Design review of the part built by this model. Coordinates are the model's own, in mm. A direction names the side the tool comes from. Coordinates: 2 decimals unless noted, no trailing zeros. Order: outer loops, then holes, each group sorted by start corner. A loop starts at its lowest first (then second) coordinate and runs counter-clockwise, first axis right, second up. Notation, with made-up numbers: M 89,4 L 109,4 A24 cw 109,25 Z; hole C -37.75,79 d1. An arc over 180 degrees is marked long. Answer as a JSON object with one key per item and string values.
from build123d import *

# Parameters (mm, degrees)
F1_DEPTH = 1.6764
F3_DEPTH = 11.938
F4_W     = 10.033
F4_H     = 5.08
F5_DEPTH = 6.5278


with BuildPart() as f1:
    # F0 (on Top) → F1 (new body)
    with BuildSketch(Plane.XY):
        Polygon((-22.5799904745, -23.241), (26.543, -23.241), (26.543, 23.241), (-22.5799904745, 23.241), (-26.543, 20.062799959), (-26.543, -20.062799959), align=None)
    extrude(amount=F1_DEPTH)

    # F2 (on face) → F3 (join)
    with BuildSketch(Plane.XY.offset(1.6764)):
        with BuildLine():
            Line((-26.543, 6.6294), (-26.543, 5.0038))
            Line((-26.543, 5.0038), (-8.255, 5.0038))
            Line((-8.255, 5.0038), (-8.255, 16.891))
            Line((-8.255, 16.891), (-26.543, 16.891))
            Line((-26.543, 16.891), (-26.543, 15.2654))
            ThreePointArc((-26.543, 15.2654), (-27.5392260553, 13.5911375004), (-26.543, 11.9168750008))
            Line((-26.543, 11.9168750008), (-26.543, 9.967618097))
            ThreePointArc((-26.543, 9.967618097), (-27.5297952384, 8.2985090485), (-26.543, 6.6294))
        make_face()
    extrude(amount=F3_DEPTH)

    # F4 (on face) → F5 (join)
    with BuildSketch(Plane(origin=(0, 0, 0), x_dir=(1, 0, 0), z_dir=(0, 0, -1))):
        with Locations((-19.9928638897, -13.5961750215)):
            Rectangle(F4_W, F4_H)
        with Locations((-19.9928638897, -6.4841750215)):
            Rectangle(F4_W, F4_H)
    extrude(amount=F5_DEPTH)


solid = f1.part
1) To check wall thickness, follow L1, parallel to Z at x = 14.5, y = 20; L2, parallel to Y at x = -9, z = 11.5; L3, parallel to X at y = -1.5, z = 1.5. State the ranges of each line that lie inside material, in increasing order.
Taken from the geometry:
{"L1": "z = 0 to 1.68", "L2": "y = 5 to 16.89", "L3": "x = -26.54 to 26.54"}
2) Mouldability with a two-part tool opening along Y and no side actions: class faces 1 (the cylindrical face through (-27.53, 8.33, 7.56)), 2 (the flat face through (2, -23.241, 1)), 3 (the flat face through (-17, 16.891, 8)) as released by +Y, released by -Y, zero draft, split by the parting line, or undercut.
Taken from the geometry:
{"face 1": "undercut", "face 2": "released by -Y", "face 3": "released by +Y"}
3) Add section C-C (y = 1). State the section outline as (x, z) points, and give its area (3 significant figures).
Taken from the geometry:
{"outline": "M -26.54,0 L 26.54,0 L 26.54,1.68 L -26.54,1.68 Z", "area": "89.0 mm2"}
4) Tool access review of faces 4 (the flat face through (-25.009, 7, -3)), 5 (the flat face through (-18, 5.004, 8)), 6 (the flat face through (-14.976, 7, -3)), 7 (the flat face through (-20, 3.944, -3)), 8 (the flat face through (-8.255, 11, 8)): name each direction out of +Z, -Z, +X, -X, +Y, -Y from which nothing blocks a thin tool from reaching the whole face with its end or side.
Taken from the geometry:
{"face 4": "-Z, -X, +Y, -Y", "face 5": "+Z, +X, -X, -Y", "face 6": "-Z, +X, +Y, -Y", "face 7": "-Z, +X, -X, -Y", "face 8": "+Z, +X, +Y, -Y"}
5) Add section A-A (z = -3.25). State the section outline as (x, y) points, and give its area (3 significant figures).
Taken from the geometry:
{"outline": "M -25.01,3.94 L -14.98,3.94 L -14.98,9.02 L -25.01,9.02 Z; M -25.01,11.06 L -14.98,11.06 L -14.98,16.14 L -25.01,16.14 Z", "area": "102 mm2"}
6) Add section D-D (z = 6.75). State the section outline as (x, y) points (1 decimal), and give its area (3 significant figures).
Taken from the geometry:
{"outline": "M -26.5,5 L -8.3,5 L -8.3,16.9 L -26.5,16.9 L -26.5,15.3 A1.9 ccw -26.5,11.9 L -26.5,10 A1.9 ccw -26.5,6.6 Z", "area": "222 mm2"}
7) Insertion check: pin 1 Ø8 at (x, y) = (12, 0.5) entering from +Z; pin 2 Ø6 at (y, z) = (8.5, 9) entering from +X (3 decimals); pin 3 Ø0.5 at (x, y) = (-27, 14.5) entering from -Z. Each pin has a flat end and moves straight along its axis. Give the tip position at first contact, or say it passes through.
Taken from the geometry:
{"pin 1": "stops at z = 1.68", "pin 2": "stops at x = -8.255", "pin 3": "stops at z = 1.68"}
8) Add section B-B (x = -13.5). State the section outline as (y, z) points, and give its area (3 significant figures).
Taken from the geometry:
{"outline": "M -23.24,0 L 23.24,0 L 23.24,1.68 L 16.89,1.68 L 16.89,13.61 L 5,13.61 L 5,1.68 L -23.24,1.68 Z", "area": "220 mm2"}
